Part model, mm, in its own coordinate system. Coordinates: 2 decimals unless noted, no trailing zeros. Loops run counter-clockwise (first coordinate to the right, second up) from the corner with the lowest first, then second, coordinate; pieces in that order, holes last. Notation, with made-up numbers: M 11.5,66 L 30.5,66 A33 cw 30.5,104 Z; hole C 8,69 d7. An arc over 180 degrees is marked long. Use a Markdown table: item, result. Add a question column.
1) Wall check: probe 1 along Y at (x, z) = (-2, 2.9); probe 2 along X at (y, z) = (254.1, 3.3); probe 3 along Y at (x, z) = (11, 5.4). Give the ranges that are in metal, low to high. Write a range as from..to.
2) Pin check, flat tips, straight feed: pin 1 Ø5 at (x, y) = (52.5, 254.1) entering from +Z; pin 2 Ø3.5 at (x, y) = (-52.3, -365.9) entering from -Z. Stop position of each tip, or through.
3) Band-saw the part on B-B (z = 2.75). State how many separate pieces and enclosed holes the cut face has, plus the area to 3 significant figures.
4) Band-saw the part on C-C (y = 306.5). List the corners of the cut face in (x, z).
5) Band-saw the part on A-A (x = 0.1). List the corners of the cut face in (y, z), plus the area to 3 significant figures.
6) Band-saw the part on D-D (x = -39.5). List the corners of the cut face in (y, z).
from build123d import *

# Parameters (mm, degrees)
ESQUISSE1_W                   = 120
ESQUISSE1_H                   = 832
BOSS_EXTRU_1_DEPTH            = 6
SKETCH1_R                     = 58.5
CUT_EXTRUDE1_DEPTH            = 10
LPATTERN1_COUNT               = 2
LPATTERN1_PITCH               = 620
M4_CLEARANCE_HOLE1_AT_2_COUNT = 2
M4_CLEARANCE_HOLE1_AT_2_PITCH = 104.8
M4_CLEARANCE_HOLE1_AT_3_COUNT = 2
M4_CLEARANCE_HOLE1_AT_3_PITCH = 148.351070101
M4_CLEARANCE_HOLE1_AT_4_COUNT = 2
M4_CLEARANCE_HOLE1_AT_4_PITCH = 104.8
LPATTERN2_COUNT               = 2
LPATTERN2_PITCH               = 620


with BuildPart() as part:
    # Esquisse1 → Boss.-Extru.1 (new body)
    with BuildSketch(Plane.XY):
        Rectangle(ESQUISSE1_W, ESQUISSE1_H)
    extrude(amount=BOSS_EXTRU_1_DEPTH)

    # Sketch1 → Cut-Extrude1 (cut)
    with BuildSketch(Plane(origin=(0, 0, 0), x_dir=(-1, 0, 0), z_dir=(0, 0, -1))):
        with Locations((-0.1, 306.5)):
            Circle(SKETCH1_R)
    cut_extrude1 = extrude(amount=-CUT_EXTRUDE1_DEPTH, mode=Mode.SUBTRACT)

    # LPattern1: Cut-Extrude1 ×2
    with Locations(*[(0, -i * LPATTERN1_PITCH, 0) for i in range(1, LPATTERN1_COUNT)]):
        add(cut_extrude1, mode=Mode.SUBTRACT)

    # Sketch2 → M4 Clearance Hole1 (revolve, cut)
    with BuildSketch(Plane(origin=(-52.3, 254.1, 0), x_dir=(0, 1, 0), z_dir=(1, 0, 0))):
        Polygon((0, 0), (0, 7.351936393), (2.25, 6), (2.25, 0), align=None)
    m4_clearance_hole1 = revolve(axis=Axis((-52.3, 254.1, -6.35), (0, 0, 1)), mode=Mode.SUBTRACT)

    # M4 Clearance Hole1 at 2: M4 Clearance Hole1 ×2
    with Locations(*[(0, i * M4_CLEARANCE_HOLE1_AT_2_PITCH, 0) for i in range(1, M4_CLEARANCE_HOLE1_AT_2_COUNT)]):
        add(m4_clearance_hole1, mode=Mode.SUBTRACT)

    # M4 Clearance Hole1 at 3: M4 Clearance Hole1 ×2
    with Locations(*[Vector(0.7077805365932406, 0.7064323831901992, 0) * (i * M4_CLEARANCE_HOLE1_AT_3_PITCH) for i in range(1, M4_CLEARANCE_HOLE1_AT_3_COUNT)]):
        add(m4_clearance_hole1, mode=Mode.SUBTRACT)

    # M4 Clearance Hole1 at 4: M4 Clearance Hole1 ×2
    with Locations(*[(i * M4_CLEARANCE_HOLE1_AT_4_PITCH, 0, 0) for i in range(1, M4_CLEARANCE_HOLE1_AT_4_COUNT)]):
        add(m4_clearance_hole1, mode=Mode.SUBTRACT)

    # LPattern2: M4 Clearance Hole1 ×2
    with Locations(*[(0, -i * LPATTERN2_PITCH, 0) for i in range(1, LPATTERN2_COUNT)]):
        add(m4_clearance_hole1, mode=Mode.SUBTRACT)

    # LPattern2 copy 1 sketch → LPattern2 copy 1 (revolve, cut)
    with BuildSketch(Plane(origin=(-52.3, -261.1, 0), x_dir=(0, 1, 0), z_dir=(1, 0, 0))):
        Polygon((0, 0), (0, 7.351936393), (2.25, 6), (2.25, 0), align=None)
    revolve(axis=Axis((-52.3, -261.1, -6.35), (0, 0, 1)), mode=Mode.SUBTRACT)

    # LPattern2 copy 2 sketch → LPattern2 copy 2 (revolve, cut)
    with BuildSketch(Plane(origin=(52.7, -261.1, 0), x_dir=(0, 1, 0), z_dir=(1, 0, 0))):
        Polygon((0, 0), (0, 7.351936393), (2.25, 6), (2.25, 0), align=None)
    revolve(axis=Axis((52.7, -261.1, -6.35), (0, 0, 1)), mode=Mode.SUBTRACT)

    # LPattern2 copy 3 sketch → LPattern2 copy 3 (revolve, cut)
    with BuildSketch(Plane(origin=(52.5, -365.9, 0), x_dir=(0, 1, 0), z_dir=(1, 0, 0))):
        Polygon((0, 0), (0, 7.351936393), (2.25, 6), (2.25, 0), align=None)
    revolve(axis=Axis((52.5, -365.9, -6.35), (0, 0, 1)), mode=Mode.SUBTRACT)


solid = part.part
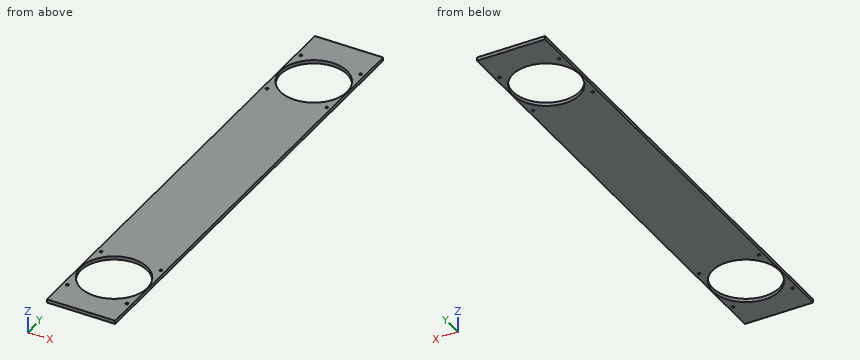
Entries:
| question | item | result |
|---|---|---|
| 1 | probe 1 | -416..-371.96, -255.04..248.04, 364.96..416 |
| 1 | probe 2 | -60..-54.55, -50.05..-25.91, 26.11..50.25, 54.75..60 |
| 1 | probe 3 | -416..-370.98, -256.02..249.02, 363.98..416 |
| 2 | pin 1 | z = 6 |
| 2 | pin 2 | through |
| 3 | separate pieces | 1 |
| 3 | enclosed holes | 10 |
| 3 | area | 78,200 mm2 |
| 4 | outline | M -60,0 L -58.4,0 L -58.4,6 L -60,6 Z; M 58.6,0 L 60,0 L 60,6 L 58.6,6 Z |
| 5 | outline | M -416,0 L -372,0 L -372,6 L -416,6 Z; M -255,0 L 248,0 L 248,6 L -255,6 Z; M 365,0 L 416,0 L 416,6 L 365,6 Z |
| 5 | area | 3,590 mm2 |
| 6 | outline | M -416,0 L -356.56,0 L -356.56,6 L -416,6 Z; M -270.44,0 L 263.44,0 L 263.44,6 L -270.44,6 Z; M 349.56,0 L 416,0 L 416,6 L 349.56,6 Z |
